Check sheet for the modelled part. Datum: model origin and axes. Units: mm. Face numbers are marked on the shaded views. A direction names the side the tool comes from. Give positions to 0.01 mm unless a question says otherwise; leave off trailing zeros. Order: outer loops, then holes, each group sorted by start corner. A loop starts at its lowest first (then second) coordinate and runs counter-clockwise, first axis right, second up.
Autodesk Inventor part; units mm, degrees
ref_plane "YZ Plane" through (0, 0, 0) normal (1, 0, 0) x (0, 1, 0)
ref_plane "XZ Plane" through (0, 0, 0) normal (0, 1, 0) x (-1, 0, 0)
ref_plane "XY Plane" through (0, 0, 0) normal (0, 0, 1) x (1, 0, 0)
sketch "Эскиз1" plane through (0, 0, 0) normal (0, 1, 0) x (-1, 0, 0)
  line L0 (0, 0) -> (21, 0)
  line L1 (21, 0) -> (21, -42)
  line L2 (21, -42) -> (0, -42)
  line L3 (0, -42) -> (0, 0)
  dimension "d0" = 21
  dimension "d1" = 42
extrude "Выдавливание1" add sketch "Эскиз1" along normal blind 1.5
sketch "Эскиз2" plane through (0, 1.5, 0) normal (0, 1, 0) x (1, 0, 0)
  line L0 (0, 0) -> (0, 42)
  line L1 (0, 39) -> (-6, 39)
  line L2 (-6, 39) -> (-6, 33)
  line L3 (-6, 33) -> (0, 33)
  line L4 (0, 33) -> (0, 39)
  line L5 (0, 42) -> (-21, 42)
  line L6 (-21, 42) -> (-21, 0)
  line L7 (-21, 3) -> (-15, 3)
  line L8 (-15, 3) -> (-15, 9)
  line L9 (-15, 9) -> (-21, 9)
  line L10 (-21, 9) -> (-21, 3)
  line L11 (-21, 0) -> (0, 0)
  point P0 (0, 33)
  dimension "d4" = 6
  dimension "d5" = 6
  dimension "d6" = 3
  dimension "d7" = 6
  dimension "d8" = 6
  dimension "d9" = 3
extrude "Выдавливание2" add sketch "Эскиз2" along normal blind 4.5 contours L3 L2 L1 L0 | L6 L9 L8 L7
fillet "Сопряжение1" radius 2 8 edges at (-15, 3.75, -3) (-15, 3.75, -9) (-6, 3.75, -33) (-6, 3.75, -39) (0, 0.75, 0) (0, 0.75, -42) (-21, 0.75, 0) (-21, 0.75, -42)
sketch "Эскиз3" plane through (0, 6, 0) normal (0, 1, 0) x (1, 0, 0)
  circle A0 centre (-18, 6) radius 0.75
  line L0 (-21, 9) -> (-21, 3)
  line L1 (-17, 9) -> (-21, 9)
  circle A1 centre (-3, 36) radius 0.75
  line L2 (0, 39) -> (-4, 39)
  line L3 (0, 33) -> (0, 39)
  point P0 (0, 0)
  dimension "d13" = 1.5
  dimension "d14" = 3
  dimension "d15" = 3
  dimension "d16" = 1.5
  dimension "d17" = 3
  dimension "d18" = 3
extrude "Выдавливание3" cut sketch "Эскиз3" against normal blind 5
properties part number "DCDC_Holder"
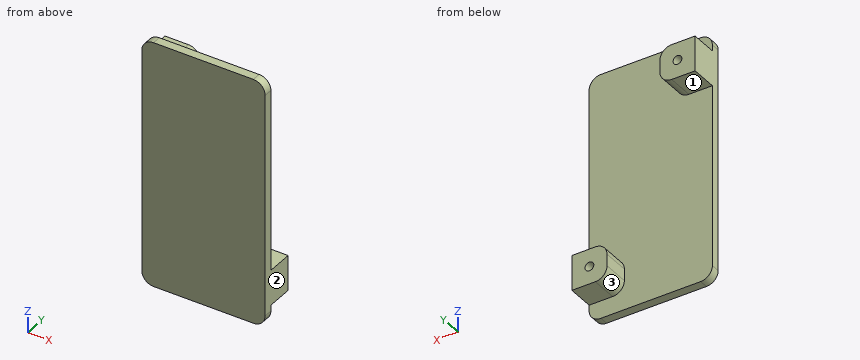
Q1. Sectioned sample at B-B, the plane x = -18. Record the cut outline in (y, z), plus the area to 3 significant figures.
Q2. Sectioned sample at D-D, the plane z = -4.5. Record the cut outline in (x, y).
Q3. Material ranges on line 1 (Z direction, x = -3, y = 3.6); line 2 (Z direction, x = -18, y = 2.5); line 3 (X direction, y = 3.35, z = -6), recorded low to high.
Q4. Sectioned sample at C-C, the plane z = -36. Record the cut outline in (x, y).
Q5. Tool access check on the marked faces 1, 2 and 3. Record the directions out of +Z, -Z, +X, -X, +Y, -Y that give a thin tool (end or side, any length) a straight path to the whole face; none if there is none.
Q6. Sectioned sample at A-A, the plane y = 3.5. Record the cut outline in (x, z).
Q7. Go/stop test with flat-tipped pins: P1, Ø1.2, axis at x = -3, y = 3.5, coming from the +Z side; P2, Ø3, axis at x = -19, y = 3.5, coming from the -Z side; P3, Ø10, axis at x = -4.5, z = -25, coming from the +Y side. Record where each tip stops, or that it passes through.
Filled in:
1. outline: (0, -42) - (1.5, -42) - (1.5, -9) - (6, -9) - (6, -6.75) - (1, -6.75) - (1, -5.25) - (6, -5.25) - (6, -3) - (1.5, -3) - (1.5, 0) - (0, 0) - close
1. area: 82.5 mm2
2. outline: (-21, 0) - (0, 0) - (0, 1.5) - (-15.06, 1.5) - (-15.06, 6) - (-21, 6) - close
3. line 1: z = -39 to -36.75, -35.25 to -33
3. line 2: z = -9 to -6.75, -5.25 to -3
3. line 3: x = -21 to -18.75, -17.25 to -15
4. outline: (-21, 0) - (0, 0) - (0, 6) - (-2.25, 6) - (-2.25, 1) - (-3.75, 1) - (-3.75, 6) - (-6, 6) - (-6, 1.5) - (-21, 1.5) - close
5. face 1: -Z, +X, -X, +Y
5. face 2: +Z, -Z, +X, +Y, -Y
5. face 3: -Z, -X, +Y
6. outline: (-21, -9) - (-17, -9) arc R2 ccw to (-15, -7) - (-15, -5) arc R2 ccw to (-17, -3) - (-21, -3) - close; (-6, -37) arc R2 ccw to (-4, -39) - (0, -39) - (0, -33) - (-4, -33) arc R2 ccw to (-6, -35) - close; hole circle Ø1.5 at (-18, -6); hole circle Ø1.5 at (-3, -36)
7. P1: stops at z = -33
7. P2: stops at z = -9
7. P3: stops at y = 1.5
